from build123d import *

# Parameters (mm, degrees)
SKETCH2_W                                  = 609.6
SKETCH2_H                                  = 609.6
BOSS_EXTRUDE1_DEPTH                        = 2.54
CUT_EXTRUDE1_DEPTH                         = 432.059777293
CUT_EXTRUDE1_DEPTH_BACK                    = 1.27
SKETCH5_R                                  = 75.5
CUT_EXTRUDE2_DEPTH                         = 432.054164694
CUT_EXTRUDE2_DEPTH_BACK                    = 432.054164694
SKETCH7_R                                  = 55
SKETCH12_R                                 = 20.123320675
BOSS_EXTRUDE2_DEPTH                        = 50
SKETCH13_R                                 = 1.5
CUT_EXTRUDE3_DEPTH                         = 10
CIRPATTERN2_COUNT                          = 6
MIRROR1_AT_THE_SECOND_PLANE_COPY_1_SKETC_R = 20.123320675
MIRROR1_AT_THE_SECOND_PLANE_COPY_1_DEPTH   = 50
SKETCH16_R                                 = 254
SKETCH16_R_2                               = 251.206
CUT_EXTRUDE6_DEPTH                         = 1.27


with BuildPart() as part:
    # Sketch2 → Boss-Extrude1 (new body)
    with BuildSketch(Plane(origin=(0, 0, 0), x_dir=(1, 0, 0), z_dir=(0, 1, 0))):
        Rectangle(SKETCH2_W, SKETCH2_H)
    extrude(amount=BOSS_EXTRUDE1_DEPTH)

    # Sketch5 → Cut-Extrude1 (cut, two sides: drawn at the far end of the back side and taken through both)
    with BuildSketch(Plane(origin=(0, 2.54, 0), x_dir=(1, 0, 0), z_dir=(0, 1, 0)).offset(-CUT_EXTRUDE1_DEPTH_BACK)):
        with Locations(Location((0, 0, 0), (0, 0, 90))):
            Circle(SKETCH5_R)
    extrude(amount=CUT_EXTRUDE1_DEPTH + CUT_EXTRUDE1_DEPTH_BACK, mode=Mode.SUBTRACT)

    # Sketch7 → Cut-Extrude2 (cut, two sides: drawn at the far end of the back side and taken through both)
    with BuildSketch(Plane(origin=(0, 1.27, 0), x_dir=(1, 0, 0), z_dir=(0, 1, 0)).offset(-CUT_EXTRUDE2_DEPTH_BACK)):
        with Locations(Location((0, 0, 0), (0, 0, 270))):
            Circle(SKETCH7_R)
    extrude(amount=CUT_EXTRUDE2_DEPTH + CUT_EXTRUDE2_DEPTH_BACK, mode=Mode.SUBTRACT)

    # Sketch12 → Boss-Extrude2 (add)
    with BuildSketch(Plane.XZ):
        with Locations(Location((-274.8, 274.8, 0), (0, 0, 270))):
            Circle(SKETCH12_R)
    boss_extrude2 = extrude(amount=BOSS_EXTRUDE2_DEPTH)

    # Sketch13 → Cut-Extrude3 (cut)
    with BuildSketch(Plane(origin=(0, 1.27, 0), x_dir=(1, 0, 0), z_dir=(0, 1, 0))):
        with Locations(Location((0, 65, 0), (0, 0, 270))):
            Circle(SKETCH13_R)
    cut_extrude3 = extrude(amount=-CUT_EXTRUDE3_DEPTH, mode=Mode.SUBTRACT)

    # CirPattern2: Cut-Extrude3 ×6 about axis
    cirpattern2_axis = Axis((0, 0, 0), (0, 1, 0))
    for i in range(1, CIRPATTERN2_COUNT):
        add(cut_extrude3.rotate(cirpattern2_axis, i * 360 / CIRPATTERN2_COUNT), mode=Mode.SUBTRACT)

    # Mirror1: Boss-Extrude2 across plane
    add(boss_extrude2.mirror(Plane.XY))

    # Mirror1 at the second plane: Boss-Extrude2 across plane
    add(boss_extrude2.mirror(Plane(origin=(0, 0, 0), x_dir=(0, 0, 1), z_dir=(1, 0, 0))))

    # Mirror1 at the second plane copy 1 sketc → Mirror1 at the second plane copy 1 (add)
    with BuildSketch(Plane(origin=(0, 0, 0), x_dir=(-1, 0, 0), z_dir=(0, -1, 0))):
        with Locations(Location((-274.8, 274.8, 0), (0, 0, 270))):
            Circle(MIRROR1_AT_THE_SECOND_PLANE_COPY_1_SKETC_R)
    extrude(amount=MIRROR1_AT_THE_SECOND_PLANE_COPY_1_DEPTH)

    # Sketch16 → Cut-Extrude6 (cut)
    with BuildSketch(Plane(origin=(0, 2.54, 0), x_dir=(1, 0, 0), z_dir=(0, 1, 0))):
        with Locations(Location((0, 0, 0), (0, 0, 270))):
            Circle(SKETCH16_R)
        with Locations(Location((0, 0, 0), (0, 0, 270))):
            Circle(SKETCH16_R_2, mode=Mode.SUBTRACT)
    extrude(amount=-CUT_EXTRUDE6_DEPTH, mode=Mode.SUBTRACT)


solid = part.part
Geometry check sheet. Reference: the model listing, model coordinates, mm. A direction names the side the tool comes from. Round coordinates to 2 decimals unless told otherwise and drop trailing zeros. Loops run counter-clockwise (first coordinate to the right, second up) from the corner with the lowest first, then second, coordinate; pieces in that order, holes last.
Item 1: Access from +Z, -Z, +X, -X, +Y, -Y to the whole of each face (thin tool, end or side, straight path). Record for faces 1 (the flat face through (-275, -50, -275)), 2 (the cylindrical face through (-222.86, 1.91, 115.92)), 3 (the cylindrical face through (-294.445, -24.65, -279.162)).
Item 2: Gauge pin test, flat end, axial feed: pin 1 (5 mm diameter, centred on x = 0, z = 65, fed in from -Y). Record the tip position at first contact, or that the pin passes through.
Item 3: Cross-section at C-C on y = -7. Record the boundary of the cut face in (x, z).
Item 4: Mould release check, pull along Z, two halves, no side actions. Record for faces 4 (the cylindrical face through (294.445, -24.65, 279.162)), 5 (the flat face through (52, 2.54, -59)): pulls with the +Z half, pulls with the -Z half, needs draft (parallel to the pull), parting line crosses it, or undercut.
Item 5: Thickness scan on line 1 (X direction, y = 1, z = 65); line 2 (X direction, y = -42, z = -276.5); line 3 (X direction, y = 0.75, z = -32.5). Record the ranges inside material, lowest first.
Item 6: Cross-section at A-A on z = 0. Record the boundary of the cut face in (x, y).
Item 7: Cross-section at B-B on x = -274.8. Record the boundary of the cut face in (y, z).
Item 8: Cross-section at D-D on z = 274.8. Record the boundary of the cut face in (x, y).
Answer sheet:
1. face 1: +Z, -Z, +X, -X, -Y
1. face 2: +Y
1. face 3: -Y
2. pin 1: stops at y = 0
3. outline: circle Ø40.25 at (-274.8, -274.8); circle Ø40.25 at (-274.8, 274.8); circle Ø40.25 at (274.8, -274.8); circle Ø40.25 at (274.8, 274.8)
4. face 4: undercut
4. face 5: needs draft
5. line 1: x = -304.8 to -1.5, 1.5 to 304.8
5. line 2: x = -294.85 to -254.75, 254.75 to 294.85
5. line 3: x = -304.8 to -57.79, -54.79 to -44.37, 44.37 to 54.79, 57.79 to 304.8
6. outline: (-304.8, 0) - (-55, 0) - (-55, 1.27) - (-75.5, 1.27) - (-75.5, 2.54) - (-251.21, 2.54) - (-251.21, 1.27) - (-254, 1.27) - (-254, 2.54) - (-304.8, 2.54) - close; (55, 0) - (304.8, 0) - (304.8, 2.54) - (254, 2.54) - (254, 1.27) - (251.21, 1.27) - (251.21, 2.54) - (75.5, 2.54) - (75.5, 1.27) - (55, 1.27) - close
7. outline: (-50, -294.92) - (0, -294.92) - (0, -304.8) - (2.54, -304.8) - (2.54, 304.8) - (0, 304.8) - (0, 294.92) - (-50, 294.92) - (-50, 254.68) - (0, 254.68) - (0, -254.68) - (-50, -254.68) - close
8. outline: (-304.8, 0) - (-294.92, 0) - (-294.92, -50) - (-254.68, -50) - (-254.68, 0) - (254.68, 0) - (254.68, -50) - (294.92, -50) - (294.92, 0) - (304.8, 0) - (304.8, 2.54) - (-304.8, 2.54) - close
